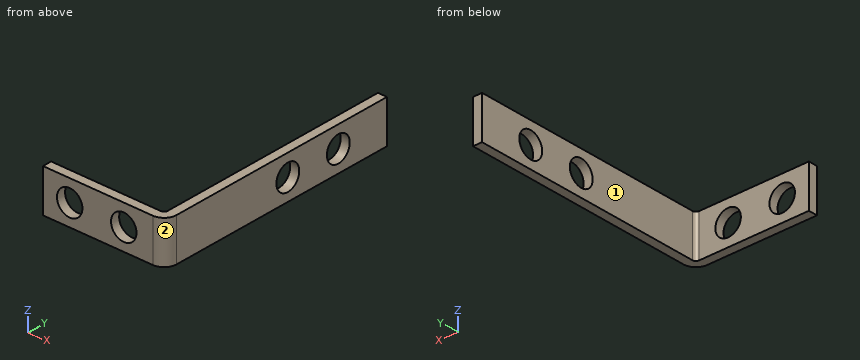
from build123d import *

# Parameters (mm, degrees)
BASE_FLANGE1_DEPTH = 7.5
SKETCH7_R          = 2.25
CUT_EXTRUDE1_DEPTH = 10
SKETCH8_R          = 2.25
CUT_EXTRUDE2_DEPTH = 10


# Sheet-metal steps are written as plain solids
with BuildPart() as part:
    # Sketch1 → Base-Flange1 (new body)
    with BuildSketch(Plane.XY):
        with BuildLine():
            Line((-20, 0), (-0.6, 0))
            ThreePointArc((-0.6, 0), (-0.175735931, 0.175735931), (0, 0.6))
            Line((0, 0.6), (0, 42))
            Line((0, 42), (1.6, 42))
            Line((1.6, 42), (1.6, 0.6))
            ThreePointArc((1.6, 0.6), (0.955634919, -0.955634919), (-0.6, -1.6))
            Line((-0.6, -1.6), (-20, -1.6))
            Line((-20, -1.6), (-20, 0))
        make_face()
    extrude(amount=BASE_FLANGE1_DEPTH)

    # Sketch7 → Cut-Extrude1 (cut)
    with BuildSketch(Plane(origin=(1.6, 0, 0), x_dir=(0, 0, -1), z_dir=(1, 0, 0))):
        with Locations((-3.75, 32.425)):
            Circle(SKETCH7_R)
        with Locations((-3.75, 22.49)):
            Circle(SKETCH7_R)
    extrude(amount=-CUT_EXTRUDE1_DEPTH, mode=Mode.SUBTRACT)

    # Sketch8 → Cut-Extrude2 (cut)
    with BuildSketch(Plane(origin=(0, 0, 0), x_dir=(1, 0, 0), z_dir=(0, 1, 0))):
        with Locations(Location((-15.288441883, -3.75, 0), (0, 0, 270))):
            Circle(SKETCH8_R)
        with Locations(Location((-5.743540806, -3.75, 0), (0, 0, 270))):
            Circle(SKETCH8_R)
    extrude(amount=-CUT_EXTRUDE2_DEPTH, mode=Mode.SUBTRACT)


solid = part.part
Work out the finished part from the listing and answer in its coordinate system (mm). Face numbers are marked on the shaded views. A direction names the side the tool comes from. Give positions to 0.01 mm unless a question says otherwise; leave off trailing zeros. Write each loop counter-clockwise with the first axis right and the second up, starting at its lowest first coordinate (ties: lowest second). Pieces come first, ordered by that corner, then holes.
Q1. The part is cut by section C-C on x = -5. Give the vertices of the cut face in (y, z).
Answer:
outline: (-1.6, 0) - (0, 0) - (0, 1.63) - (-1.6, 1.63) - close; (-1.6, 5.87) - (0, 5.87) - (0, 7.5) - (-1.6, 7.5) - close
Q2. The part is cut by section B-B on y = 22.49. Give the vertices of the cut face in (x, z).
Answer:
outline: (0, 0) - (1.6, 0) - (1.6, 1.5) - (0, 1.5) - close; (0, 6) - (1.6, 6) - (1.6, 7.5) - (0, 7.5) - close
Q3. A tool of negligible diameter and unlimited length cuts with its end or side. For the marked faces 1 and 2, from which of +Z, -Z, +X, -X, +Y, -Y can it reach the whole face along a straight path? Write none if from no direction.
Answer:
face 1: +Z, -Z, -X, +Y
face 2: +Z, -Z, +X, -Y
Q4. The part is cut by section A-A on z = 3.75. Give the vertices of the cut face in (x, y) (3 decimals).
Answer:
outline: (-20, -1.6) - (-17.538, -1.6) - (-17.538, 0) - (-20, 0) - close; (-13.038, -1.6) - (-7.994, -1.6) - (-7.994, 0) - (-13.038, 0) - close; (-3.494, -1.6) - (-0.6, -1.6) arc R2.2 ccw to (1.6, 0.6) - (1.6, 20.24) - (0, 20.24) - (0, 0.6) arc R0.6 cw to (-0.6, 0) - (-3.494, 0) - close; (0, 24.74) - (1.6, 24.74) - (1.6, 30.175) - (0, 30.175) - close; (0, 34.675) - (1.6, 34.675) - (1.6, 42) - (0, 42) - close
Q5. Given pin 1 (2 mm diameter, centred on x = -15.5, z = 5.5, fed in from +Y), flat-ended and moving along its own axis, determine where the tip first touches the part or whether it passes through.
Answer:
pin 1: stops at y = 0
Q6. Straight lines are drawn through the part: L1, parallel to Y at x = 1.25, z = 3.75 (3 decimals); L2, parallel to X at y = -0.95, z = 3.75; L3, parallel to X at y = -1.2, z = 3.75. For each, find the intervals that lie inside material, in ascending order.
Answer:
L1: y = -0.591 to 20.24, 24.74 to 30.175, 34.675 to 42
L2: x = -20 to -17.54, -13.04 to -7.99, -3.49 to 0.96
L3: x = -20 to -17.54, -13.04 to -7.99, -3.49 to 0.66
Q7. The part is cut by section D-D on z = 6.5. Give the vertices of the cut face in (x, y), and give its area (3 significant figures).
Answer:
outline: (-20, -1.6) - (-0.6, -1.6) arc R2.2 ccw to (1.6, 0.6) - (1.6, 42) - (0, 42) - (0, 0.6) arc R0.6 cw to (-0.6, 0) - (-20, 0) - close
area: 101 mm2
